Source: CAD feature listing. Evaluate the final solid. Frame: model axes, mm. A direction names the side the tool comes from. Round coordinates to 2 decimals unless told otherwise and drop trailing zeros. Order: outer loops, then holes, each group sorted by start corner. A loop starts at its lowest first (then second) coordinate and runs counter-clockwise, first axis right, second up. Notation, with made-up numbers: M 61,33.5 L 119,33.5 A19 ccw 119,43.5 Z; hole C 5.25,14.25 d7. An arc over 180 degrees is marked long. Use one line per item in the form item = value. Start each with the question number.
Q1. Section C-C (x = 3.5). Return the cut outline in (y, z).
Q2. Contact query for flat-ended pins moving along their axis: pin 1 (4 mm diameter, centred on x = 12, z = 11, fed in from +Y); pin 2 (6 mm diameter, centred on y = 6.5, z = 4, fed in from -X); pin 3 (4.5 mm diameter, centred on x = 24, y = 7, fed in from +Z); pin 4 (3 mm diameter, centred on x = -12, z = 11, fed in from +Y). Output: stop coordinate, or through.
Q3. Section B-B (z = 11). Return the cut outline in (x, y).
Q4. Section A-A (x = -12). Return the cut outline in (y, z).
Q5. Material intervals for probe 1 along Z at (x, y) = (-12, 2.25); probe 2 along Z at (x, y) = (12, 4); probe 3 along X at (y, z) = (2, 12), sorted ascending.
Q6. Section D-D (y = 4.5). Give the number of separate pieces and of enclosed holes in the cut face, plus the area to 3 significant figures.
Q7. Reachability of faces 4 (the flat face through (23, 6, 10)), 5 (the flat face through (-10.6, 3, 9.6)), 6 (the flat face through (0, 6, 7)) from +Z, -Z, +X, -X, +Y, -Y: full face, straight path, thin tool, end or side. Return the list, or none.
Q8. Pull-direction query (Z, two-part tool) for faces 1 (the cylindrical face through (-13.524, 4.521, 10.368)), 2 (the flat face through (-23, 6, 10)), 3 (the cylindrical face through (27.27, 0.29, 3.14)); classes: pulls with the +Z half, pulls with the -Z half, needs draft (parallel to the pull), parting line crosses it, or undercut.
from build123d import *

# Parameters (mm, degrees)
F1_DEPTH       = 10
F2_W           = 34
F2_H           = 6
F3_DEPTH       = 5
F5_R           = 2.49999
F6_D           = 3.3
F6_CBORE_D     = 6.5
F6_CBORE_DEPTH = 3
F7_T1_DEPTH    = 28.1801488287
F7_T3_DEPTH    = 28.1801488287
F8_R           = 1.65
F9_DEPTH       = 49.9246466694
F10_R          = 1.65
F11_DEPTH      = 49.9246466694
F13_R          = 3.25
F14_DEPTH      = 25
F16_R          = 3.25
F17_DEPTH      = 25


# Not quite as in the source:
# - a fillet or chamfer that OpenCascade refuses, or shapes differently, is made with other operations: its cross-section is extruded or revolved along the edge and cut away or added
# - a fillet or chamfer is up to 0.001 mm smaller than in the source, because OpenCascade refuses the exact size


with BuildPart() as f1:
    # F0 (on Top) → F1 (new body)
    with BuildSketch(Plane.XY):
        with BuildLine():
            Line((-25.5868655417, 0), (0, 0))
            Line((0, 0), (25.5868655417, 0))
            ThreePointArc((25.5868655417, 0), (27.2969662583, 0.3015368961), (28.8008035901, 1.1697777844))
            Line((28.8008035901, 1.1697777844), (31.2369389286, 3.2139380484))
            Line((31.2369389286, 3.2139380484), (24.8090628318, 10.8743824796))
            Line((24.8090628318, 10.8743824796), (20.3940868771, 7.1697777844))
            ThreePointArc((20.3940868771, 7.1697777844), (18.8902495453, 6.3015368961), (17.1801488287, 6))
            Line((17.1801488287, 6), (0, 6))
            Line((0, 6), (-17.1801488287, 6))
            ThreePointArc((-17.1801488287, 6), (-18.8902495453, 6.3015368961), (-20.3940868771, 7.1697777844))
            Line((-20.3940868771, 7.1697777844), (-24.8090628318, 10.8743824796))
            Line((-24.8090628318, 10.8743824796), (-31.2369389286, 3.2139380484))
            Line((-31.2369389286, 3.2139380484), (-28.8008035901, 1.1697777844))
            ThreePointArc((-28.8008035901, 1.1697777844), (-27.2969662583, 0.3015368961), (-25.5868655417, 0))
        make_face()
    extrude(amount=F1_DEPTH)

    # F2 (on face) → F3 (join)
    with BuildSketch(Plane.XY.offset(10)):
        with Locations((0, 3)):
            Rectangle(F2_W, F2_H)
    extrude(amount=F3_DEPTH)

    # F5 (radius 2.5 in the source; OpenCascade refuses exactly that, so slightly less here)
    f5_edges = [f1.edges().sort_by_distance(p)[0] for p in [
        (17, 3, 10),
        (17, 3, 15),
        (-17, 3, 15),
        (-17, 3, 10),
    ]]
    fillet(f5_edges, radius=F5_R)

    # F6 (through all)
    with Locations(Plane.XZ):
        with Locations((-12, 11), (12, 11)):
            CounterBoreHole(F6_D / 2, F6_CBORE_D / 2, F6_CBORE_DEPTH)

    # F7: fillet of radius 5 on 2 edges, made by hand

    # F7_s2 → F7_t1 (cut)
    with BuildSketch(Plane(origin=(-29.4886993176, 24.7439567213, 0), x_dir=(0, 0, 1), z_dir=(0.7660444431, -0.6427876097, 0))):
        with BuildLine():
            ThreePointArc((10, 12.6166979253), (8.5355339059, 16.1522318313), (5, 17.6166979253))
            Line((5, 17.6166979253), (10, 17.6166979253))
            Line((10, 17.6166979253), (10, 12.6166979253))
        make_face()
    extrude(amount=F7_T1_DEPTH, mode=Mode.SUBTRACT)

    # F7_s4 → F7_t3 (cut)
    with BuildSketch(Plane(origin=(7.9014529012, 6.6301062151, 0), x_dir=(0, 0, 1), z_dir=(0.7660444431, 0.6427876097, 0))):
        with BuildLine():
            ThreePointArc((5, 17.6166979253), (8.5355339059, 16.1522318313), (10, 12.6166979253))
            Line((10, 12.6166979253), (10, 17.6166979253))
            Line((10, 17.6166979253), (5, 17.6166979253))
        make_face()
    extrude(amount=F7_T3_DEPTH, mode=Mode.SUBTRACT)

    # F8 (on face) → F9 (cut, through all)
    with BuildSketch(Plane(origin=(19.9131437786, 16.7091116002, 0), x_dir=(-0.6427876097, 0.7660444431, 0), z_dir=(0.7660444431, 0.6427876097, 0))):
        with Locations((-12.6166979253, 5)):
            Circle(F8_R)
    extrude(amount=-F9_DEPTH, mode=Mode.SUBTRACT)

    # F10 (on face) → F11 (cut, through all)
    with BuildSketch(Plane(origin=(-19.9131437786, 16.7091116002, 0), x_dir=(-0.6427876097, -0.7660444431, 0), z_dir=(-0.7660444431, 0.6427876097, 0))):
        with Locations((12.6166979253, 5)):
            Circle(F10_R)
    extrude(amount=-F11_DEPTH, mode=Mode.SUBTRACT)

    # F13 (on offset) → F14 (cut)
    with BuildSketch(Plane(origin=(16.082921563, 13.4951735518, 0), x_dir=(-0.6427876097, 0.7660444431, 0), z_dir=(0.7660444431, 0.6427876097, 0))):
        with Locations((-12.6, 5)):
            Circle(F13_R)
    extrude(amount=-F14_DEPTH, mode=Mode.SUBTRACT)

    # F16 (on offset) → F17 (cut)
    with BuildSketch(Plane(origin=(-16.082921563, 13.4951735518, 0), x_dir=(-0.6427876097, -0.7660444431, 0), z_dir=(-0.7660444431, 0.6427876097, 0))):
        with Locations((12.6, 5)):
            Circle(F16_R)
    extrude(amount=-F17_DEPTH, mode=Mode.SUBTRACT)


solid = f1.part
Results list:
q1.outline = M 0,0 L 6,0 L 6,15 L 0,15 Z
q2.pin_1 = 6
q2.pin_2 = -31
q2.pin_3 = 10
q2.pin_4 = through
q3.outline = M -17.5,0 L -15.25,0 L -15.25,3 L -13.65,3 L -13.65,6 L -17.18,6 A5 cw -17.5,6.01 Z; M -10.35,3 L -8.75,3 L -8.75,0 L 8.75,0 L 8.75,3 L 10.35,3 L 10.35,6 L -10.35,6 Z; M 13.65,3 L 15.25,3 L 15.25,0 L 17.5,0 L 17.5,6.01 A5 cw 17.18,6 L 13.65,6 Z
q4.outline = M 0,0 L 6,0 L 6,9.35 L 3,9.35 L 3,7.75 L 0,7.75 Z; M 0,14.25 L 3,14.25 L 3,12.65 L 6,12.65 L 6,15 L 0,15 Z
q5.probe_1 = 0 to 7.75, 14.25 to 15
q5.probe_2 = 0 to 9.35, 12.65 to 15
q5.probe_3 = -17.05 to -15.09, -8.91 to 8.91, 15.09 to 17.05
q6.separate_pieces = 1
q6.enclosed_holes = 4
q6.area = 696 mm2
q7.face_4 = +Z, +X, +Y, -Y
q7.face_5 = -Y
q7.face_6 = +Z, -Z, +Y
q8.face_1 = undercut
q8.face_2 = pulls with the +Z half
q8.face_3 = needs draft
